```python
from build123d import *

# Parameters (mm, degrees)
F0_R         = 3
F1_DEPTH     = 4
F0_R_2       = 3.4
F2_DEPTH     = 10
F3_SIZE      = 1
F4_T1_DEPTH  = 22.1100533903
F4_T3_DEPTH  = 10
F4_T10_DEPTH = 44.4806964521
F4_S11_R     = 7.5
F4_T12_DEPTH = 24
F4_T14_ANGLE = 90
F4_T18_DEPTH = 44.4806964521
F4_S19_R     = 7.5
F4_T20_DEPTH = 24
F4_T22_ANGLE = 90


# Not quite as in the source:
# - a fillet or chamfer that OpenCascade refuses, or shapes differently, is made with other operations: its cross-section is extruded or revolved along the edge and cut away or added


with BuildPart() as f1:
    # F0 (on Top) → F1 (new body)
    with BuildSketch(Plane.XY):
        with BuildLine():
            Line((10, -34.3899466097), (7.5, 0))
            ThreePointArc((7.5, 0), (0, -7.5), (-7.5, 0))
            Line((-7.5, 0), (-10, -34.3899466097))
            Line((-10, -34.3899466097), (-10, -54))
            ThreePointArc((-10, -54), (-8.5355339059, -57.5355339059), (-5, -59))
            Line((-5, -59), (5, -59))
            ThreePointArc((5, -59), (8.5355339059, -57.5355339059), (10, -54))
            Line((10, -54), (10, -34.3899466097))
        make_face()
        with Locations((0, -49)):
            Circle(F0_R, mode=Mode.SUBTRACT)
        with Locations((0, -34)):
            Circle(F0_R, mode=Mode.SUBTRACT)
    extrude(amount=F1_DEPTH)

    # F0 (on Top) → F2 (join)
    with BuildSketch(Plane.XY):
        with BuildLine():
            ThreePointArc((-7.5, 0), (0, -7.5), (7.5, 0))
            ThreePointArc((7.5, 0), (0, 7.5), (-7.5, 0))
        make_face()
        Circle(F0_R_2, mode=Mode.SUBTRACT)
    extrude(amount=F2_DEPTH)

    # F3
    f3_edges = [f1.edges().sort_by_distance(p)[0] for p in [
        (-3, -34, 4),
        (-3, -49, 4),
        (-3.4, 0, 10),
    ]]
    chamfer(f3_edges, length=F3_SIZE)

    # F4: fillet of radius 1 on 5 edges, made by hand

    # F4_s2 → F4_t1 (cut)
    with BuildSketch(Plane.XZ.offset(31.8899466097)):
        with BuildLine():
            ThreePointArc((-9, 4), (-9.7071067812, 3.7071067812), (-10, 3))
            Line((-10, 3), (-10, 4))
            Line((-10, 4), (-9, 4))
        make_face()
        with BuildLine():
            ThreePointArc((9, 4), (9.7071067812, 3.7071067812), (10, 3))
            Line((10, 3), (10, 4))
            Line((10, 4), (9, 4))
        make_face()
    extrude(amount=F4_T1_DEPTH, mode=Mode.SUBTRACT)

    # F4_s4 → F4_t3 (cut)
    with BuildSketch(Plane.YZ.offset(-5)):
        with BuildLine():
            ThreePointArc((-58, 4), (-58.7071067812, 3.7071067812), (-59, 3))
            Line((-59, 3), (-59, 4))
            Line((-59, 4), (-58, 4))
        make_face()
    extrude(amount=F4_T3_DEPTH, mode=Mode.SUBTRACT)

    # F4_s5 → F4_t6 (revolve, cut)
    with BuildSketch(Plane.XZ):
        with BuildLine():
            ThreePointArc((7.5, 9), (7.2071067812, 9.7071067812), (6.5, 10))
            Line((6.5, 10), (7.5, 10))
            Line((7.5, 10), (7.5, 9))
        make_face()
    revolve(axis=Axis((0, 0, 10), (0, 0, -1)), mode=Mode.SUBTRACT)


with BuildPart() as f4_tool8:
    # F4_s9 → F4_t10 (new body)
    with BuildSketch(Plane(origin=(0.5043559293, 6.9379093918, 0), x_dir=(0, 0, 1), z_dir=(-0.072504336, -0.9973680972, 0))):
        with BuildLine():
            ThreePointArc((4, 6.4802607288), (3.7071067812, 7.18736751), (3, 7.4802607288))
            Line((3, 7.4802607288), (4, 7.4802607288))
            Line((4, 7.4802607288), (4, 6.4802607288))
        make_face()
    extrude(amount=F4_T10_DEPTH)

    # F4_s11 → F4_t12 (cut, symmetric)
    with BuildSketch(Plane.XY.offset(3.5)):
        Circle(F4_S11_R)
    extrude(amount=F4_T12_DEPTH, both=True, mode=Mode.SUBTRACT)


with BuildPart() as f1_1:
    add(f1.part)

    # F4_t7: cut F4_tool8
    add(f4_tool8.part, mode=Mode.SUBTRACT)

    # F4_s13 → F4_t14 (revolve, cut)
    with BuildSketch(Plane.XZ.offset(54)):
        with BuildLine():
            ThreePointArc((-9, 4), (-9.7071067812, 3.7071067812), (-10, 3))
            Line((-10, 3), (-10, 4))
            Line((-10, 4), (-9, 4))
        make_face()
    revolve(axis=Axis((-5, -54, 4), (0, 0, 1)), revolution_arc=F4_T14_ANGLE, mode=Mode.SUBTRACT)


with BuildPart() as f4_tool16:
    # F4_s17 → F4_t18 (new body)
    with BuildSketch(Plane(origin=(2.7206874304, -37.4257181897, 0), x_dir=(0, 0, 1), z_dir=(-0.072504336, 0.9973680972, 0))):
        with BuildLine():
            ThreePointArc((4, 6.4802607288), (3.7071067812, 7.18736751), (3, 7.4802607288))
            Line((3, 7.4802607288), (4, 7.4802607288))
            Line((4, 7.4802607288), (4, 6.4802607288))
        make_face()
    extrude(amount=F4_T18_DEPTH)

    # F4_s19 → F4_t20 (cut, symmetric)
    with BuildSketch(Plane.XY.offset(3.5)):
        Circle(F4_S19_R)
    extrude(amount=F4_T20_DEPTH, both=True, mode=Mode.SUBTRACT)


with BuildPart() as f1_2:
    add(f1_1.part)

    # F4_t15: cut F4_tool16
    add(f4_tool16.part, mode=Mode.SUBTRACT)

    # F4_s21 → F4_t22 (revolve, cut)
    with BuildSketch(Plane.YZ.offset(5)):
        with BuildLine():
            ThreePointArc((-58, 4), (-58.7071067812, 3.7071067812), (-59, 3))
            Line((-59, 3), (-59, 4))
            Line((-59, 4), (-58, 4))
        make_face()
    revolve(axis=Axis((5, -54, 4), (0, 0, 1)), revolution_arc=F4_T22_ANGLE, mode=Mode.SUBTRACT)


solid = f1_2.part
```
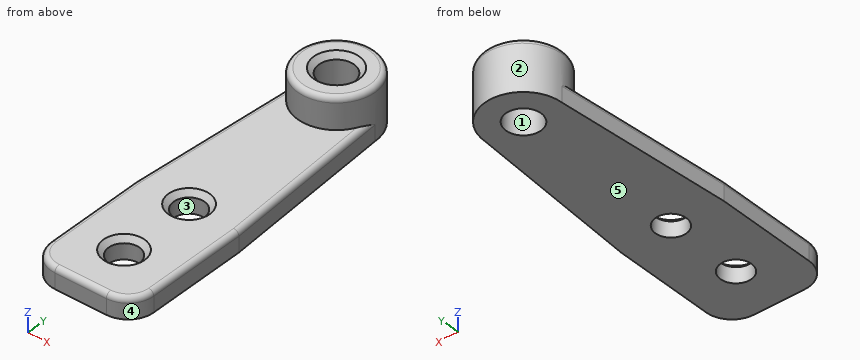
Can you work these out from the model? Positions are in its coordinate system, mm. Face numbers are marked on the shaded views. A direction names the side the tool comes from. Coordinates: 2 decimals unless noted, no trailing zeros. Loops run counter-clockwise (first coordinate to the right, second up) from the corner with the lowest first, then second, coordinate; pieces in that order, holes last. Notation, with made-up numbers: M 18,67 L 47,67 A15 cw 47,86 Z; hole C 7,-33 d9. An arc over 180 degrees is marked long. Put each result on its own line as item: value. Start each with the question number.
(1) Which directions (+Z, -Z, +X, -X, +Y, -Y) give clear straight access to the entire face, cutting with the end or side of a thin tool? Please do the marked faces 1 and 2.
(2) Imagine slicing it at B-B on z = 1.5. List the corners of the cut face in (x, y) for me, and give its area (3 significant figures).
(3) Imagine slicing it at D-D on z = 7. List the corners of the cut face in (x, y) for me.
(4) Imagine slicing it at C-C on y = -49. List the corners of the cut face in (x, z) for me.
(5) Imagine slicing it at A-A on x = 0. List the corners of the cut face in (y, z) for me, and give its area (3 significant figures).
(6) We'd pull the mould along Y, two halves only. Please class the marked faces 3, 4 and 5: +Y half, -Y half, draft (parallel to the pull), parting line (faces both ways), or undercut.
(7) Will these pins go through, and if not, where does the flat tip stop? pin 1 Ø4 at (x, y) = (-6.5, -16) entering from +Z; pin 2 Ø6 at (x, z) = (1, 7.5) entering from -Y; pin 3 Ø1.5 at (y, z) = (-2, 1.5) entering from -X.
(8) I need wall thicknesses on probe 1 along Y at (x, z) = (0, 0.8); probe 2 along Y at (x, z) = (-3.75, 4.75); probe 3 along Z at (x, y) = (-4, -11). Which ranges of each line are inside material? Lowest first, please.
Worked answers:
1. face 1: +Z, -Z
1. face 2: +Z
2. outline: M -10,-54 A5 ccw -5,-59 L 5,-59 A5 ccw 10,-54 L 10,-34.39 L 7.5,0 A7.5 ccw -7.5,0 L -10,-34.39 Z; hole C 0,0 d6.8; hole C 0,-49 d6; hole C 0,-34 d6
2. area: 1,080 mm2
3. outline: C 0,0 d15; hole C 0,0 d6.8
4. outline: M -10,0 L -3,0 L -3,3 L -4,4 L -9,4 A1 ccw -10,3 Z; M 3,0 L 10,0 L 10,3 A1 ccw 9,4 L 4,4 L 3,3 Z
5. outline: M -59,0 L -52,0 L -52,3 L -53,4 L -58,4 A1 ccw -59,3 Z; M -46,0 L -37,0 L -37,3 L -38,4 L -45,4 L -46,3 Z; M -31,0 L -3.4,0 L -3.4,9 L -4.4,10 L -6.5,10 A1 ccw -7.5,9 L -7.5,4 L -30,4 L -31,3 Z; M 3.4,0 L 7.5,0 L 7.5,9 A1 ccw 6.5,10 L 4.4,10 L 3.4,9 Z
5. area: 236 mm2
6. face 3: undercut
6. face 4: -Y half
6. face 5: draft
7. pin 1: stops at z = 4
7. pin 2: stops at y = -7.5
7. pin 3: stops at x = -7.7
8. probe 1: y = -59 to -52, -46 to -37, -31 to -3.4, 3.4 to 7.5
8. probe 2: y = -6.5 to 6.5
8. probe 3: z = 0 to 4
